Geometry check sheet. Reference: the model listing, model coordinates, mm. Face numbers are marked on the shaded views. A direction names the side the tool comes from. Coordinates: 2 decimals unless noted, no trailing zeros. Write each loop counter-clockwise with the first axis right and the second up, starting at its lowest first coordinate (ties: lowest second). Pieces come first, ordered by that corner, then holes. Notation, with made-up numbers: (24, -28.75) -> (82, -28.75) arc R20 ccw to (82, -5.75) -> close; hole circle Ø1 at (69, 56.25). An arc over 180 degrees is marked (long way). One line per question, with ' | ' between items.
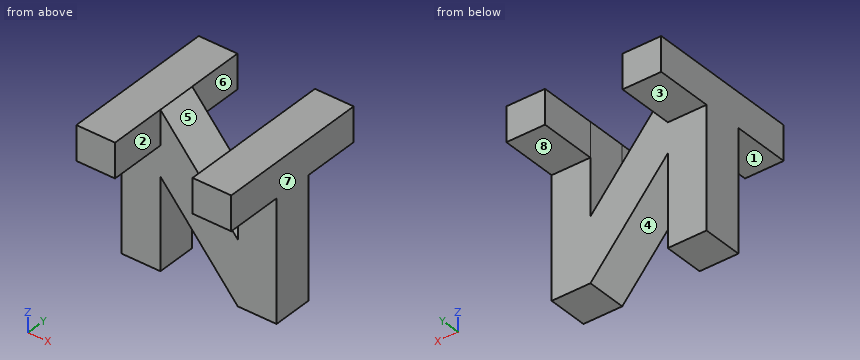
```python
from build123d import *

# Parameters (mm, degrees)
F0_W     = 25.4
F0_H     = 25.4
F1_DEPTH = 25.4
F5_DEPTH = 25.401
F6_DEPTH = 25.401
F7_DEPTH = 25.401


with BuildPart() as f1:
    # F0 (on Top) → F1 (new body)
    with BuildSketch(Plane.XY):
        Rectangle(F0_W, F0_H)
    extrude(amount=F1_DEPTH)

    # F2 (on face) → F5 (intersect, through all)
    with BuildSketch(Plane.XY.offset(25.4)):
        Polygon((-6.357004, 12.7), (-12.7, 12.7), (-12.7, -12.7), (-6.357004, -12.7), (-6.357004, -3.302), (0, -3.302), (6.357004, -3.302), (6.357004, -12.7), (12.7, -12.7), (12.7, 12.7), (6.357004, 12.7), (6.357004, 3.302), (0, 3.302), (-6.357004, 3.302), align=None)
    extrude(amount=-F5_DEPTH, mode=Mode.INTERSECT)

    # F3 (on face) → F6 (intersect, through all)
    with BuildSketch(Plane(origin=(-12.7, 0, 0), x_dir=(0, -1, 0), z_dir=(-1, 0, 0))):
        Polygon((0, 25.4), (-12.7, 25.4), (-12.7, 19.764362), (-3.302, 19.764362), (-3.302, 0), (0, 0), (3.302, 0), (3.302, 19.764362), (12.7, 19.764362), (12.7, 25.4), align=None)
    extrude(amount=-F6_DEPTH, mode=Mode.INTERSECT)

    # F4 (on face) → F7 (intersect, through all)
    with BuildSketch(Plane.XZ.offset(12.7)):
        Polygon((-6.340738, 25.4), (-12.7, 25.4), (-12.7, 0), (-6.340738, 0), (-6.340738, 14.896067), (6.340738, 0), (12.7, 0), (12.7, 25.4), (6.340738, 25.4), (6.340738, 10.503933), align=None)
    extrude(amount=-F7_DEPTH, mode=Mode.INTERSECT)


solid = f1.part
```
(1) Material ranges on line 1 (X direction, y = 7.5, z = 23.25); line 2 (X direction, y = 0.25, z = 13.5); line 3 (Y direction, x = 4.5, z = 6.25), recorded low to high.
Answers below:
line 1: x = -12.7 to -6.36, 6.36 to 12.7 | line 2: x = -12.7 to -6.34, -5.15 to 3.79, 6.34 to 12.7 | line 3: y = -3.3 to 3.3
(2) Cross-section at A-A (y = 5.5). Record the cut outline in (x, z).
Answers below:
outline: (-12.7, 19.76) -> (-6.36, 19.76) -> (-6.36, 25.4) -> (-12.7, 25.4) -> close; (6.36, 19.76) -> (12.7, 19.76) -> (12.7, 25.4) -> (6.36, 25.4) -> close
(3) Cross-section at B-B (z = 15.25). Record the cut outline in (x, y).
Answers below:
outline: (-12.7, -3.3) -> (2.3, -3.3) -> (2.3, 3.3) -> (-12.7, 3.3) -> close; (6.34, -3.3) -> (12.7, -3.3) -> (12.7, 3.3) -> (6.34, 3.3) -> close
(4) Cross-section at C-C (x = 9). Record the cut outline in (y, z), plus the area to 3 significant figures.
Answers below:
outline: (-12.7, 19.76) -> (-3.3, 19.76) -> (-3.3, 0) -> (3.3, 0) -> (3.3, 19.76) -> (12.7, 19.76) -> (12.7, 25.4) -> (-12.7, 25.4) -> close | area: 274 mm²
(5) Depth check by flat-ended pin: P1, Ø1, axis at x = -3.5, z = 17.5, coming from the -Y side; P2, Ø5, axis at x = 8.5, y = -7, coming from the -Z side; P3, Ø7.5, axis at x = 1, z = 10, coming from the +Y side; P4, Ø1, axis at x = 5.5, y = 4, coming from the -Z side. Enter the tip coordinate at first touch or a pass-through.
Answers below:
P1: stops at y = -3.3 | P2: stops at z = 19.76 | P3: stops at y = 3.3 | P4: passes through
(6) Draft check along X on the marked faces 5, 6, 7 and 8. Enter one of: pulls with the +X half, pulls with the -X half, needs draft (parallel to the pull), parting line crosses it, or undercut.
Answers below:
face 5: undercut | face 6: undercut | face 7: pulls with the +X half | face 8: needs draft
(7) Tool access check on the marked faces 1, 2, 3 and 4. Record the directions out of +Z, -Z, +X, -X, +Y, -Y that give a thin tool (end or side, any length) a straight path to the whole face; none if there is none.
Answers below:
face 1: -Z, +X, -X, -Y | face 2: +Z, -Z, -Y | face 3: -Z, +X, -X, +Y | face 4: -Z, +Y, -Y
